Here's how the part is built. I have some questions about the finished solid (model axes, mm). A direction names the side the tool comes from. Give positions to 0.01 mm unless a question says otherwise; leave off trailing zeros. Write each loop counter-clockwise with the first axis right and the second up, starting at its lowest first coordinate (ties: lowest second). Pieces come first, ordered by that corner, then holes. Notation, with made-up numbers: (70, 79.25) - (76, 79.25) arc R11 cw to (76, 84.25) - close; hole circle Ø5 at (87, -24.75). An arc over 180 degrees is marked (long way). Write each question's results on one line, items separated by ' | '. Start each with the question number.
Item 1: We'd pull the mould along X, two halves only. Please class faces 1 (the flat face through (-1.8, 13, -3.4)), 2 (the flat face through (-4, -0.2, 3.3)), 3 (the cylindrical face through (-2.44, -0.54, 10.12)), 4 (the cylindrical face through (-1.341, 3.233, 13.138)): +X half, -X half, draft (parallel to the pull), parting line (faces both ways), or undercut.
Item 2: Suppose I cut it at D-D on y = 10.5. List the corners of the cut face in (x, z) for me.
Item 3: Which directions (+Z, -Z, +X, -X, +Y, -Y) give clear straight access to the entire face, cutting with the end or side of a thin tool? Please do faces 5 (the cylindrical face through (-0.54, -9.12, 2.44)), 6 (the cylindrical face through (0, -3, 0)), 7 (the cylindrical face through (-1.341, -3.233, -13.138)), 8 (the flat face through (-2, 2, 12.3)), 9 (the cylindrical face through (-0.54, 9.12, -2.44)).
Item 4: Suppose I cut it at A-A on z = 0. List the corners of the cut face in (x, y) for me, then the cut area to 3 significant figures.
Item 5: Suppose I cut it at B-B on y = 0. List the corners of the cut face in (x, z) for me.
Item 6: Please list where these lines run through material, in increasing order: line 1 along X through (y, z) = (0, -13); line 2 along Z through (x, y) = (-3, 0); line 3 along Y through (x, z) = (2, -0.5).
Item 7: Suppose I cut it at C-C on z = 9. List the corners of the cut face in (x, y) for me, then the cut area to 3 significant figures.
Item 8: Will these pins go through, and if not, where does the flat tip stop? P1, Ø1.5, axis at x = 3, y = 8.5, coming from the -Z side; P2, Ø5, axis at y = 0, z = 0, coming from the +X side; P3, Ø2.5, axis at x = -0.5, y = -1, coming from the +Z side; P4, Ø4, axis at x = 0, z = 0, coming from the -Y side.
Autodesk Inventor part; units mm, degrees
ref_plane "YZ Plane" through (0, 0, 0) normal (1, 0, 0) x (0, 1, 0)
ref_plane "XZ Plane" through (0, 0, 0) normal (0, 1, 0) x (-1, 0, 0)
ref_plane "XY Plane" through (0, 0, 0) normal (0, 0, 1) x (1, 0, 0)
sketch "草圖4" plane through (0, 0, 0) normal (1, 0, 0) x (0, 1, 0)
  line L0 (4, 14) -> (-4, 14)
  line L1 (-13, 5) -> (-13, -5)
  line L2 (-4, -14) -> (4, -14)
  line L3 (13, -5) -> (13, 5)
  arc A0 (13, 5) -> (4, 14) centre (4, 5) ccw
  arc A1 (4, -14) -> (13, -5) centre (4, -5) ccw
  arc A2 (-13, -5) -> (-4, -14) centre (-4, -5) ccw
  arc A3 (-4, 14) -> (-13, 5) centre (-4, 5) ccw
  circle A4 centre (0, 0) radius 3
  point P0 (-13, -14)
  point P1 (-13, 14)
  point P2 (13, -14)
  point P3 (0, 14)
  point P4 (13, 0)
  dimension "d13" = 26
  dimension "d14" = 28
  dimension "d15" = 9
  dimension "d23" = 6
extrude "擠出1" add sketch "草圖4" along normal mid plane 8
sketch "草圖3" plane through (0, 0, 0) normal (0, 0, 1) x (1, 0, 0)
  line L0 (0, 13) -> (3.5, 13)
  line L1 (3.5, 13) -> (3.5, 11.3)
  line L2 (3.5, 11.3) -> (2.5, 11.3)
  line L3 (2.5, 11.3) -> (2.5, 7)
  line L4 (2.5, 7) -> (0, 7)
  line L5 (0, 13) -> (0, 7)
  line L6 (4, 13) -> (-4, 13) construction
  point P0 (0, 0)
  dimension "d5" = 1.7
  dimension "d6" = 7
  dimension "d7" = 6
  dimension "d8" = 5
revolve "迴轉2" cut sketch "草圖3" angle 360 about axis through (0, 13, 0) along (0, -1, 0)
sketch "草圖5" plane through (0, 0, 0) normal (1, 0, 0) x (0, 1, 0)
  line L0 (0, 14) -> (3.5, 14)
  line L1 (3.5, 14) -> (3.5, 12.3)
  line L2 (3.5, 12.3) -> (2.5, 12.3)
  line L3 (2.5, 12.3) -> (2.5, 8)
  line L4 (2.5, 8) -> (0, 8)
  line L5 (0, 14) -> (0, 8)
  line L6 (-4, 14) -> (4, 14) construction
  point P0 (0, 0)
  point P1 (0, 0)
  dimension "d18" = 1.7
  dimension "d19" = 7
  dimension "d20" = 6
  dimension "d21" = 5
revolve "迴轉3" cut sketch "草圖5" angle 360 about axis through (0, 0, 14) along (0, 0, -1)
pattern_circular "環形陣列1" count 2 over 360 about axis through (-10, 0, 0) along (1, 0, 0) of "迴轉2", "迴轉3"
properties part number "限位塊" material "SS41"
Checked values:
1) face 1: draft | face 2: -X half | face 3: undercut | face 4: undercut
2) outline: (-4, -11.22) - (4, -11.22) - (4, 11.22) - (-4, 11.22) - close; hole circle Ø5 at (0, 0)
3) face 5: -Y | face 6: +X, -X | face 7: -Z | face 8: +Z | face 9: +Y
4) outline: (-4, -13) - (-3.5, -13) - (-3.5, -11.3) - (-2.5, -11.3) - (-2.5, -7) - (2.5, -7) - (2.5, -11.3) - (3.5, -11.3) - (3.5, -13) - (4, -13) - (4, -3) - (-4, -3) - close; (-4, 3) - (4, 3) - (4, 13) - (3.5, 13) - (3.5, 11.3) - (2.5, 11.3) - (2.5, 7) - (-2.5, 7) - (-2.5, 11.3) - (-3.5, 11.3) - (-3.5, 13) - (-4, 13) - close | area: 93.2 mm^2
5) outline: (-4, -14) - (-3.5, -14) - (-3.5, -12.3) - (-2.5, -12.3) - (-2.5, -8) - (2.5, -8) - (2.5, -12.3) - (3.5, -12.3) - (3.5, -14) - (4, -14) - (4, -3) - (-4, -3) - close; (-4, 3) - (4, 3) - (4, 14) - (3.5, 14) - (3.5, 12.3) - (2.5, 12.3) - (2.5, 8) - (-2.5, 8) - (-2.5, 12.3) - (-3.5, 12.3) - (-3.5, 14) - (-4, 14) - close
6) line 1: x = -4 to -3.5, 3.5 to 4 | line 2: z = -12.3 to -3, 3 to 12.3 | line 3: y = -7 to -2.96, 2.96 to 7
7) outline: (-4, -12.06) - (4, -12.06) - (4, 12.06) - (-4, 12.06) - close; hole circle Ø5 at (0, 0) | area: 173 mm^2
8) P1: stops at z = -13.18 | P2: passes through | P3: stops at z = 8 | P4: stops at y = -7
